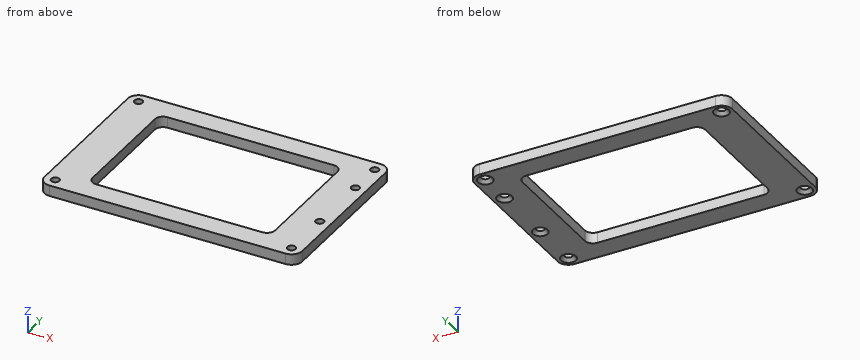
```python
from build123d import *

# Parameters (mm, degrees)
F0_R     = 2.413
F1_DEPTH = 6.35
F2_SIZE  = 1.9812
F3_SIZE  = 1.9812


with BuildPart() as f1:
    # F0 (on Top) → F1 (new body)
    with BuildSketch(Plane.XY):
        with BuildLine():
            ThreePointArc((-76.2, -44.45), (-74.340128, -48.940128), (-69.85, -50.8))
            Line((-69.85, -50.8), (69.85, -50.8))
            ThreePointArc((69.85, -50.8), (74.340128, -48.940128), (76.2, -44.45))
            Line((76.2, -44.45), (76.2, 44.45))
            ThreePointArc((76.2, 44.45), (74.340128, 48.940128), (69.85, 50.8))
            Line((69.85, 50.8), (-69.85, 50.8))
            ThreePointArc((-69.85, 50.8), (-74.340128, 48.940128), (-76.2, 44.45))
            Line((-76.2, 44.45), (-76.2, -44.45))
        make_face()
        with Locations((-69.85, -44.45)):
            Circle(F0_R, mode=Mode.SUBTRACT)
        with Locations((69.85, -44.45)):
            Circle(F0_R, mode=Mode.SUBTRACT)
        with Locations((69.85, -14.2748)):
            Circle(F0_R, mode=Mode.SUBTRACT)
        with Locations((-69.85, 44.45)):
            Circle(F0_R, mode=Mode.SUBTRACT)
        with BuildLine():
            ThreePointArc((-53.975, 33.3248), (-52.576376, 36.701376), (-49.1998, 38.1))
            Line((-49.1998, 38.1), (49.1998, 38.1))
            ThreePointArc((49.1998, 38.1), (52.576376, 36.701376), (53.975, 33.3248))
            Line((53.975, 33.3248), (53.975, -33.3248))
            ThreePointArc((53.975, -33.3248), (52.576376, -36.701376), (49.1998, -38.1))
            Line((49.1998, -38.1), (-49.1998, -38.1))
            ThreePointArc((-49.1998, -38.1), (-52.576376, -36.701376), (-53.975, -33.3248))
            Line((-53.975, -33.3248), (-53.975, 33.3248))
        make_face(mode=Mode.SUBTRACT)
        with Locations((69.85, 23.8125)):
            Circle(F0_R, mode=Mode.SUBTRACT)
        with Locations((69.85, 44.45)):
            Circle(F0_R, mode=Mode.SUBTRACT)
    extrude(amount=F1_DEPTH)

    # F2
    f2_edges = [f1.edges().sort_by_distance(p)[0] for p in [
        (-72.263, 44.45, 0),
        (-72.263, -44.45, 0),
        (67.437, 44.45, 0),
        (67.437, -44.45, 0),
    ]]
    chamfer(f2_edges, length=F2_SIZE)

    # F3
    f3_edges = [f1.edges().sort_by_distance(p)[0] for p in [
        (67.437, 23.8125, 0),
        (67.437, -14.2748, 0),
    ]]
    chamfer(f3_edges, length=F3_SIZE)


solid = f1.part
```
Input: part model. Units: mm. Frame: model coordinates. Round coordinates to 2 decimals unless told otherwise and drop trailing zeros. Order: outer loops, then holes, each group sorted by start corner. A loop starts at its lowest first (then second) coordinate and runs counter-clockwise, first axis right, second up. Notation, with made-up numbers: (-6, 38) - (49, 38) arc R29 ccw to (49, 63) - close; hole circle Ø5 at (11, 87). An arc over 180 degrees is marked (long way). One line per question, with ' | ' between items. Start each with the question number.
1) Contact query for flat-ended pins moving along their axis: P1, Ø6.5, axis at x = 69.85, y = 23.81, coming from the -Z side; P2, Ø4, axis at x = 69.85, y = -44.45, coming from the +Z side; P3, Ø5.5, axis at x = -69.85, y = -44.45, coming from the -Z side. Output: stop coordinate, or through.
2) Cut plane B-B, the plane x = 27. Return the cut outline in (y, z).
3) Cut plane A-A, the plane y = -30. Return the cut outline in (x, z) (3 decimals).
4) Ray query, probe 1 along Y at (x, z) = (69.85, 5); probe 2 along Y at (x, z) = (-69.85, 4.5); probe 3 along Y at (x, z) = (-20, 4.5). Return the intervals inside material, ascending.
Worked out:
1) P1: stops at z = 1.14 | P2: passes through | P3: stops at z = 1.64
2) outline: (-50.8, 0) - (-38.1, 0) - (-38.1, 6.35) - (-50.8, 6.35) - close; (38.1, 0) - (50.8, 0) - (50.8, 6.35) - (38.1, 6.35) - close
3) outline: (-76.2, 0) - (-53.975, 0) - (-53.975, 6.35) - (-76.2, 6.35) - close; (53.975, 0) - (76.2, 0) - (76.2, 6.35) - (53.975, 6.35) - close
4) probe 1: y = -50.8 to -46.86, -42.04 to -16.69, -11.86 to 21.4, 26.23 to 42.04, 46.86 to 50.8 | probe 2: y = -50.8 to -46.86, -42.04 to 42.04, 46.86 to 50.8 | probe 3: y = -50.8 to -38.1, 38.1 to 50.8
